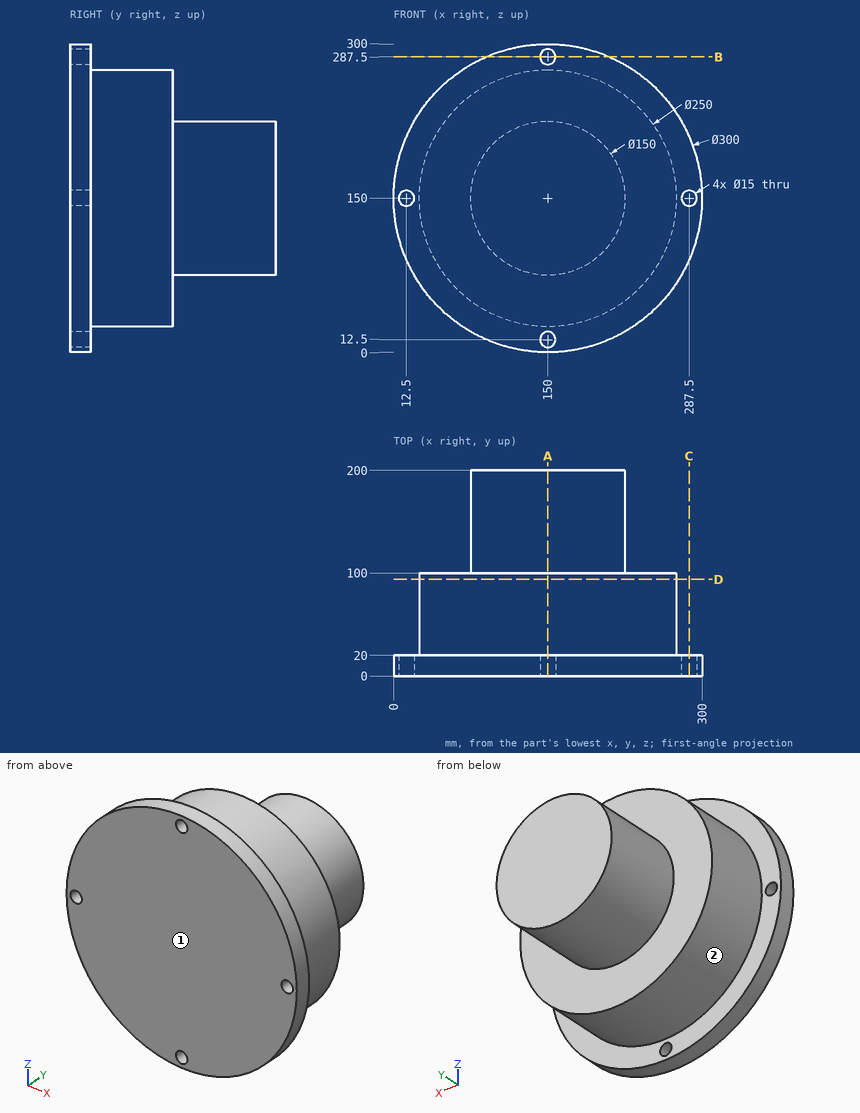
The figure shows three views and two pictorial views of one solid part (mm, origin at its lowest corner). Answer the questions. A direction names the side the tool comes from. Coordinates: 2 decimals unless noted, no trailing zeros. Loops run counter-clockwise (first coordinate to the right, second up) from the corner with the lowest first, then second, coordinate; pieces in that order, holes last. Notation, with made-up numbers: (-34, -22) - (-5, -22) arc R35 ccw to (-5, 17) - close; hole circle Ø10 at (39.25, -2). An arc over 180 degrees is marked (long way). Use a Markdown table: item, result. Add a question column.
1) Find the intervals of material crossed by line 1 (X direction, y = 15.5, z = 150); line 2 (Y direction, x = 20, z = 152); line 3 (X direction, y = 5.5, z = 287.5), in increasing order.
2) For the marked faces 1 and 2, determine the directions among +Z, -Z, +X, -X, +Y, -Y from which every point of the face is accessible in a straight line to the end or side of a thin tool.
3) Given pin 1 (19.5 mm diameter, centred on x = 287.5, z = 150, fed in from +Y); pin 2 (10 mm diameter, centred on y = 99.5, z = 184, fed in from +X); pin 3 (1.5 mm diameter, centred on x = 166.5, z = 50.5, fed in from +Y), each flat-ended and moving along its own axis, determine where each tip first touches the part or whether it passes through.
4) The part is cut by section D-D, the plane y = 94. Give the vertices of the cut face in (x, z), and give its area (3 significant figures).
5) The part is cut by section B-B, the plane z = 287.5. Give the vertices of the cut face in (x, y), and give its area (3 significant figures).
6) The part is cut by section C-C, the plane x = 287.5. Give the vertices of the cut face in (y, z), and give its area (3 significant figures).
7) The part is cut by section A-A, the plane x = 150. Give the vertices of the cut face in (y, z), and give its area (3 significant figures).
Here are the results:
| question | item | result |
|---|---|---|
| 1 | line 1 | x = 0 to 5, 20 to 280, 295 to 300 |
| 1 | line 2 | y = 0 to 20 |
| 1 | line 3 | x = 90.05 to 142.5, 157.5 to 209.95 |
| 2 | face 1 | +Z, -Z, +X, -X, -Y |
| 2 | face 2 | +Y |
| 3 | pin 1 | stops at y = 20 |
| 3 | pin 2 | stops at x = 271.59 |
| 3 | pin 3 | stops at y = 100 |
| 4 | outline | circle Ø250 at (150, 150) |
| 4 | area | 49,100 mm^2 |
| 5 | outline | (90.05, 0) - (142.5, 0) - (142.5, 20) - (90.05, 20) - close; (157.5, 0) - (209.95, 0) - (209.95, 20) - (157.5, 20) - close |
| 5 | area | 2,100 mm^2 |
| 6 | outline | (0, 90.05) - (20, 90.05) - (20, 142.5) - (0, 142.5) - close; (0, 157.5) - (20, 157.5) - (20, 209.95) - (0, 209.95) - close |
| 6 | area | 2,100 mm^2 |
| 7 | outline | (0, 0) - (20, 0) - (20, 5) - (0, 5) - close; (0, 20) - (20, 20) - (20, 25) - (100, 25) - (100, 75) - (200, 75) - (200, 225) - (100, 225) - (100, 275) - (20, 275) - (20, 280) - (0, 280) - close; (0, 295) - (20, 295) - (20, 300) - (0, 300) - close |
| 7 | area | 40,400 mm^2 |
